Geometry: final body of the model. Coordinates: model frame, mm. A direction names the side the tool comes from. Give positions to 0.01 mm unless a question says otherwise; leave off trailing zeros. Order: outer loops, then holes, each group sorted by start corner. A loop starts at its lowest first (then second) coordinate and runs counter-clockwise, first axis right, second up. Notation, with made-up numbers: (66.25, 54.5) - (78.25, 54.5) arc R13 cw to (78.25, 70.5) - close; hole circle Ø6 at (-1.5, -11.5). An arc over 180 degrees is marked (long way). Write item = value, one per line. Start each with the question number.
from build123d import *

# Parameters (mm, degrees)
SKETCH1_R                = 43.18
SKETCH1_R_2              = 35.56
BOSS_EXTRUDE1_DEPTH      = 5.08
SKETCH1_4_R              = 49.53
SKETCH1_4_R_2            = 43.18
BOSS_EXTRUDE2_DEPTH      = 12.7
BOSS_EXTRUDE3_DEPTH      = 12.7
SKETCH3_W                = 10.16
SKETCH3_H                = 6.35
BOSS_EXTRUDE4_DEPTH      = 90.932
SKETCH4_R                = 4.495372053
BOSS_EXTRUDE5_DEPTH      = 43.18
BOSS_EXTRUDE5_DEPTH_BACK = 8.89


with BuildPart() as part:
    # Sketch1 → Boss-Extrude1 (new body)
    with BuildSketch(Plane.XY):
        Circle(SKETCH1_R)
        Circle(SKETCH1_R_2, mode=Mode.SUBTRACT)
    extrude(amount=-BOSS_EXTRUDE1_DEPTH)

    # Sketch1_4 → Boss-Extrude2 (add)
    with BuildSketch(Plane.XY):
        Circle(SKETCH1_4_R)
        Circle(SKETCH1_4_R_2, mode=Mode.SUBTRACT)
    extrude(amount=-BOSS_EXTRUDE2_DEPTH)

    # Sketch2 → Boss-Extrude3 (add)
    with BuildSketch(Plane.XY):
        with BuildLine():
            ThreePointArc((49.53, 0), (0, -49.53), (-49.53, 0))
            Line((-49.53, 0), (-49.53, -49.53))
            Line((-49.53, -49.53), (-49.53, -86.36))
            Line((-49.53, -86.36), (0, -86.36))
            Line((0, -86.36), (49.53, -86.36))
            Line((49.53, -86.36), (49.53, 0))
        make_face()
    extrude(amount=-BOSS_EXTRUDE3_DEPTH)

    # Sketch3 → Boss-Extrude4 (add)
    with BuildSketch(Plane.ZY.offset(49.53)):
        with Locations((-17.78, -83.185)):
            Rectangle(SKETCH3_W, SKETCH3_H)
    extrude(amount=-BOSS_EXTRUDE4_DEPTH)

    # Sketch4 → Boss-Extrude5 (add, two sides)
    with BuildSketch(Plane(origin=(0, 0, -12.7), x_dir=(-1, 0, 0), z_dir=(0, 0, -1))) as boss_extrude5_sk:
        with Locations((-17.696483248, -36.755496611)):
            Circle(SKETCH4_R)
        with Locations((20.052531589, -36.755496611)):
            Circle(SKETCH4_R)
    extrude(amount=BOSS_EXTRUDE5_DEPTH)
    extrude(boss_extrude5_sk.sketch, amount=-BOSS_EXTRUDE5_DEPTH_BACK)


solid = part.part
Q1. Material intervals for line 1 along Y through (x, z) = (0, -8.5); line 2 along X through (y, z) = (0, -6); line 3 along Y through (x, z) = (0, -3.05), sorted ascending. Write a range as from..to.
Q2. Set-up query: faces 4 (the flat face through (41.402, -83, -18)), 5 (the flat face through (-20, -37, -55.88)). Return all of +Z, -Z, +X, -X, +Y, -Y with unobstructed straight access to the full face (end or side cutting, diameter ignored); none if empty.
Q3. Section B-B, the plane z = -8. Return the cut outline in (x, y), then the cut area to 3 significant figures.
Q4. Section C-C, the plane y = 15. Return the cut outline in (x, z), then the cut area to 3 significant figures.
Q5. Section A-A, the plane x = 0. Return the cut outline in (y, z), then the cut area to 3 significant figures.
Q6. Pull-direction query (X, two-part tool) for faces 1 (the flat face through (6.2, 35.4, -5.08)), 2 (the cylindrical face through (1.09, 49.52, -6.26)), 3 (the flat face through (-5, -83, -22.86)); classes: +X half, -X half, draft (parallel to the pull), parting line (faces both ways), or undercut.
Q7. Contact query for flat-ended pins moving along their axis: pin 1 (3 mm diameter, centred on y = -84, z = -17, fed in from +X); pin 2 (3 mm diameter, centred on x = 5.5, z = -17.5, fed in from +Y); pin 3 (2 mm diameter, centred on x = -39.5, y = -39.5, fed in from -Z); pin 4 (2 mm diameter, centred on x = -23, y = -54, fed in from +Z). Output: stop coordinate, or through.
Q8. Section D-D, the plane z = -19.5. Return the cut outline in (x, y).
The answers:
q1.line_1 = -86.36..-43.18, 43.18..49.53
q1.line_2 = -49.53..-43.18, 43.18..49.53
q1.line_3 = -86.36..-35.56, 35.56..49.53
q2.face_4 = -Z, +X, +Y, -Y
q2.face_5 = -Z, +X, -X, +Y, -Y
q3.outline = (-49.53, -86.36) - (49.53, -86.36) - (49.53, 0) arc R49.53 ccw to (-49.53, 0) - close; hole (-24.4, -35.62) arc R4.5 cw (long way) to (-16.75, -39.8) arc R43.18 ccw to (15.13, -40.44) arc R4.5 cw (long way) to (22.18, -37.05) arc R43.18 ccw (long way) to start
q3.area = 6,650 mm²
q4.outline = (-47.2, -12.7) - (-40.49, -12.7) - (-40.49, -5.08) - (-32.24, -5.08) - (-32.24, 0) - (-47.2, 0) - close; (32.24, -5.08) - (40.49, -5.08) - (40.49, -12.7) - (47.2, -12.7) - (47.2, 0) - (32.24, 0) - close
q4.area = 254 mm²
q5.outline = (-86.36, -22.86) - (-80.01, -22.86) - (-80.01, -12.7) - (-43.18, -12.7) - (-43.18, -5.08) - (-35.56, -5.08) - (-35.56, 0) - (-86.36, 0) - close; (35.56, -5.08) - (43.18, -5.08) - (43.18, -12.7) - (49.53, -12.7) - (49.53, 0) - (35.56, 0) - close
q5.area = 771 mm²
q6.face_1 = undercut
q6.face_2 = parting line
q6.face_3 = draft
q7.pin_1 = 41.4
q7.pin_2 = -80.01
q7.pin_3 = -12.7
q7.pin_4 = 0
q8.outline = (-49.53, -86.36) - (41.4, -86.36) - (41.4, -80.01) - (-49.53, -80.01) - close; circle Ø8.99 at (-20.05, -36.76); circle Ø8.99 at (17.7, -36.76)
